```python
from build123d import *

# Parameters (mm, degrees)
CUT_EXTRUDE_1_DEPTH = 2
FILLET_1_R          = 0.1


with BuildPart() as part:
    # 草图1 → 旋转1 (revolve)
    with BuildSketch(Plane.XY, mode=Mode.PRIVATE) as revolve_1_sk:
        Polygon((0, 0), (0, 11), (2.8, 11), (2.8, 8), (1.5, 8), (1.5, 0), align=None)
    revolve(revolve_1_sk.sketch.rotate(Axis((0, 0, 0), (0, 1, 0)), 90), axis=Axis((0, 0, 0), (0, 1, 0)))

    # 草图2 → 切除-拉伸1 (cut)
    with BuildSketch(Plane(origin=(0, 11, 0), x_dir=(1, 0, 0), z_dir=(0, 1, 0))):
        Polygon((1.075295482, -0.962846281), (1.37149708, 0.449810063), (0.296201598, 1.412656344), (-1.075295482, 0.962846281), (-1.37149708, -0.449810063), (-0.296201598, -1.412656344), align=None)
    extrude(amount=-CUT_EXTRUDE_1_DEPTH, mode=Mode.SUBTRACT)

    # 圆角1
    fillet_1_edges = [part.edges().sort_by_distance(p)[0] for p in [
        (0, 8, 2.8),
        (0, 11, 2.8),
    ]]
    fillet(fillet_1_edges, radius=FILLET_1_R)


solid = part.part
```
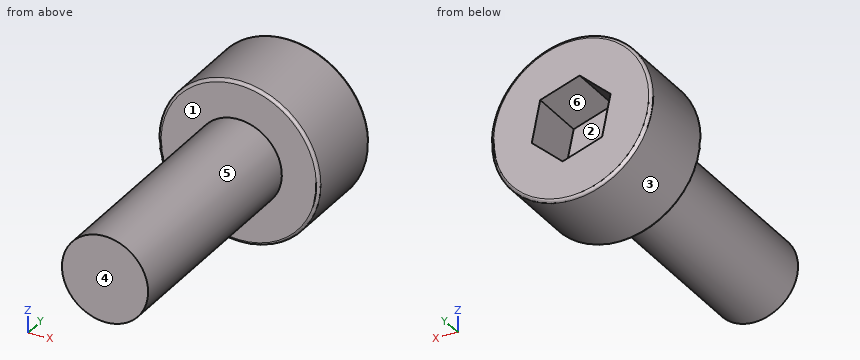
Read the model definition and answer for the solid it produces. Units are mm, in the model's axes. Face numbers are marked on the shaded views. A direction names the side the tool comes from. Give positions to 0.01 mm unless a question says otherwise; leave off trailing zeros. Write each loop counter-clockwise with the first axis right and the second up, starting at its lowest first coordinate (ties: lowest second). Pieces come first, ordered by that corner, then holes. Notation, with made-up numbers: (-1.5, 70.5) -> (31.5, 70.5) arc R19 ccw to (31.5, 105.5) -> close; hole circle Ø1 at (40.5, 63). An arc over 180 degrees is marked (long way). Answer as a JSON object with one key per item and string values.
1) For a pull along X with two mould halves and no side action, classify the marked faces 1, 2 and 3 as pulls with the +X half, pulls with the -X half, needs draft (parallel to the pull), parting line crosses it, or undercut.
Findings below:
{"face 1": "needs draft", "face 2": "undercut", "face 3": "parting line crosses it"}
2) Section B-B on x = 0 is taken. Write down the section's boundary in (y, z), then the cut area to 3 significant figures.
Findings below:
{"outline": "(0, -1.5) -> (8, -1.5) -> (8, -2.7) arc R0.1 ccw to (8.1, -2.8) -> (10.9, -2.8) arc R0.1 ccw to (11, -2.7) -> (11, -1.32) -> (9, -1.32) -> (9, 1.32) -> (11, 1.32) -> (11, 2.7) arc R0.1 ccw to (10.9, 2.8) -> (8.1, 2.8) arc R0.1 ccw to (8, 2.7) -> (8, 1.5) -> (0, 1.5) -> close", "area": "35.5 mm^2"}
3) Section A-A on y = 9.75 is taken. Write down the section's boundary in (x, z).
Findings below:
{"outline": "circle Ø5.6 at (0, 0); hole (-1.37, 0.45) -> (-1.08, -0.96) -> (0.3, -1.41) -> (1.37, -0.45) -> (1.08, 0.96) -> (-0.3, 1.41) -> close"}
4) Section D-D on z = 0 is taken. Write down the section's boundary in (x, y), then the cut area to 3 significant figures.
Findings below:
{"outline": "(-2.8, 8.1) arc R0.1 ccw to (-2.7, 8) -> (-1.5, 8) -> (-1.5, 0) -> (1.5, 0) -> (1.5, 8) -> (2.7, 8) arc R0.1 ccw to (2.8, 8.1) -> (2.8, 10.9) arc R0.1 ccw to (2.7, 11) -> (1.28, 11) -> (1.28, 9) -> (-1.28, 9) -> (-1.28, 11) -> (-2.7, 11) arc R0.1 ccw to (-2.8, 10.9) -> close", "area": "35.7 mm^2"}
5) A tool of negligible diameter and unlimited length cuts with its end or side. For the marked faces 4, 5 and 6, from which of +Z, -Z, +X, -X, +Y, -Y can it reach the whole face along a straight path? Write none if from no direction.
Findings below:
{"face 4": "+Z, -Z, +X, -X, -Y", "face 5": "-Y", "face 6": "+Y"}
6) A flat-ended cylindrical pin translates along its axis: pin 1 Ø1 at (x, y) = (0.5, 5) entering from +Z. Find the tip coordinate at first contact, or state that the pin passes through.
Findings below:
{"pin 1": "stops at z = 1.5"}
7) Section C-C on y = 3 is taken. Write down the section's boundary in (x, z), then the cut area to 3 significant figures.
Findings below:
{"outline": "circle Ø3 at (0, 0)", "area": "7.07 mm^2"}
8) Straight lines are drawn through the part: probe 1 along Y at (x, z) = (-1.55, 1.6); probe 2 along Z at (x, y) = (-0.5, 7.75); probe 3 along Z at (x, y) = (0.1, 3.5). For each, find the intervals that lie inside material, in ascending order. Write a range as from..to.
Findings below:
{"probe 1": "y = 8..11", "probe 2": "z = -1.41..1.41", "probe 3": "z = -1.5..1.5"}
